Could you check a few things on this model? Use its own coordinates, in mm. A direction names the side the tool comes from. Give positions to 0.01 mm unless a question says otherwise; leave off trailing zeros. Loops run counter-clockwise (first coordinate to the right, second up) from the corner with the lowest first, then second, coordinate; pieces in that order, holes last. Notation, with made-up numbers: M 14.5,56.5 L 31.5,56.5 A23 cw 31.5,69.5 Z; hole C 27,52.5 d4. An arc over 180 degrees is marked long. Use a Markdown table: item, result. Add a question column.
1) Suppose I cut it at B-B on z = -1.25. List the corners of the cut face in (x, y) for me.
2) If I drill on line 1 along Y through (x, z) = (0.25, 2); line 2 along Y through (x, z) = (0, -1.5); line 3 along Y through (x, z) = (-2.25, -0.75), over which ranges is the centre line in solid material (lowest first)? Write a range as [from, to].
3) Suppose I cut it at A-A on x = 0. List the corners of the cut face in (y, z) for me.
4) Suppose I cut it at C-C on y = -8. List the corners of the cut face in (x, z) for me, and give its area (3 significant figures).
5) Will these pins go through, and if not, where does the flat tip stop? pin 1 Ø3 at (x, y) = (0, 25.01) entering from -Z; pin 2 Ø3 at (x, y) = (0, -5) entering from +Z; pin 3 Ø1 at (x, z) = (2.5, 0) entering from +Y.
6) Which directions (+Z, -Z, +X, -X, +Y, -Y) give clear straight access to the entire face, cutting with the end or side of a thin tool? Please do faces 1 (the flat face through (-2, 0, 2)), 2 (the cylindrical face through (-0.728, 57.605, -1.755)), 3 (the flat face through (-3.5, 25, 0)).
7) We'd pull the mould along Y, two halves only. Please class faces 4 (the cylindrical face through (-0.728, -7.395, -1.755)), 5 (the flat face through (0, -15, 0)), 6 (the flat face through (-2, 50, 2)), 7 (the cylindrical face through (-0.434, 23.058, 0.049)): +Y half, -Y half, draft (parallel to the pull), parting line (faces both ways), or undercut.
```python
from build123d import *

# Parameters (mm, degrees)
SKETCH2_W                = 7
SKETCH2_H                = 7
BOSS_EXTRUDE1_DEPTH      = 50
BOSS_EXTRUDE3_DEPTH      = 15
BOSS_EXTRUDE3_DEPTH_BACK = 65
SKETCH3_R                = 1.9
SKETCH4_R                = 2
CUT_EXTRUDE1_DEPTH       = 10


with BuildPart() as part:
    # Sketch2 → Boss-Extrude1 (new body)
    with BuildSketch(Plane(origin=(0, 0, 0), x_dir=(1, 0, 0), z_dir=(0, 1, 0))):
        Rectangle(SKETCH2_W, SKETCH2_H)
    extrude(amount=BOSS_EXTRUDE1_DEPTH)

    # Sketch3 → Boss-Extrude3 (add, two sides: drawn at the far end of the back side and taken through both)
    with BuildSketch(Plane.XZ.offset(-BOSS_EXTRUDE3_DEPTH_BACK)):
        with Locations(Location((0, 0, 0), (0, 0, 270))):
            Circle(SKETCH3_R)
    extrude(amount=BOSS_EXTRUDE3_DEPTH + BOSS_EXTRUDE3_DEPTH_BACK)

    # Sketch4 → Cut-Extrude1 (cut)
    with BuildSketch(Plane.XY.offset(3.5)):
        with Locations((0, 25.010433152)):
            Circle(SKETCH4_R)
    extrude(amount=-CUT_EXTRUDE1_DEPTH, mode=Mode.SUBTRACT)


solid = part.part
```
Answer block:
| question | item | result |
|---|---|---|
| 1 | outline | M -3.5,0 L -1.43,0 L -1.43,-15 L 1.43,-15 L 1.43,0 L 3.5,0 L 3.5,50 L 1.43,50 L 1.43,65 L -1.43,65 L -1.43,50 L -3.5,50 Z; hole C 0,25.01 d4 |
| 2 | line 1 | y = [0, 23.03], [26.99, 50] |
| 2 | line 2 | y = [-15, 23.01], [27.01, 65] |
| 2 | line 3 | y = [0, 50] |
| 3 | outline | M -15,-1.9 L 0,-1.9 L 0,-3.5 L 23.01,-3.5 L 23.01,3.5 L 0,3.5 L 0,1.9 L -15,1.9 Z; M 27.01,-3.5 L 50,-3.5 L 50,-1.9 L 65,-1.9 L 65,1.9 L 50,1.9 L 50,3.5 L 27.01,3.5 Z |
| 4 | outline | C 0,0 d3.8 |
| 4 | area | 11.3 mm^2 |
| 5 | pin 1 | passes through |
| 5 | pin 2 | stops at z = 1.9 |
| 5 | pin 3 | stops at y = 50 |
| 6 | face 1 | -Y |
| 6 | face 2 | +Y |
| 6 | face 3 | +Z, -Z, -X, +Y, -Y |
| 7 | face 4 | draft |
| 7 | face 5 | -Y half |
| 7 | face 6 | +Y half |
| 7 | face 7 | undercut |
